from build123d import *

# Parameters (mm, degrees)
SKETCH1_W           = 25.25
SKETCH1_H           = 16
BOSS_EXTRUDE1_DEPTH = 1.7
BOSS_EXTRUDE3_DEPTH = 12.625
CUT_EXTRUDE7_DEPTH  = 9.75
CUT_EXTRUDE8_REACH  = 21.549


with BuildPart() as part:
    # Sketch1 → Boss-Extrude1 (new body)
    with BuildSketch(Plane(origin=(0, 0, 0), x_dir=(1, 0, 0), z_dir=(0, 1, 0))):
        Rectangle(SKETCH1_W, SKETCH1_H)
    extrude(amount=BOSS_EXTRUDE1_DEPTH)

    # Sketch5 → Boss-Extrude3 (add, symmetric)
    with BuildSketch(Plane(origin=(0, 0, 0), x_dir=(0, 0, -1), z_dir=(1, 0, 0))):
        Polygon((-8, 1.7), (8, 1.7), (8, 12.6), (5, 12.6), (-8, 5), align=None)
    extrude(amount=BOSS_EXTRUDE3_DEPTH, both=True)

    # Sketch5<2> → Cut-Extrude7 (cut, symmetric)
    with BuildSketch(Plane(origin=(0, 0, 0), x_dir=(0, 0, -1), z_dir=(1, 0, 0))):
        Polygon((-8, 1.7), (8, 1.7), (8, 12.6), (5, 12.6), (-8, 5), align=None)
    extrude(amount=CUT_EXTRUDE7_DEPTH, both=True, mode=Mode.SUBTRACT)

    # Sketch6 → Cut-Extrude8 (cut, up to next)
    with BuildSketch(Plane(origin=(0, 0, 0), x_dir=(1, 0, 0), z_dir=(0, 1, 0)), mode=Mode.PRIVATE) as cut_extrude8_sk1:
        with BuildLine():
            Line((-5.125, -2.5), (-2.325, -2.5))
            ThreePointArc((-2.325, -2.5), (-0.825, -4), (-2.325, -5.5))
            Line((-2.325, -5.5), (-5.125, -5.5))
            ThreePointArc((-5.125, -5.5), (-6.625, -4), (-5.125, -2.5))
        make_face()
    cut_extrude8_tool1 = extrude(cut_extrude8_sk1.sketch, amount=CUT_EXTRUDE8_REACH, mode=Mode.PRIVATE) & part.part
    # Sketch6 → Cut-Extrude8 (cut, up to next)
    with BuildSketch(Plane(origin=(0, 0, 0), x_dir=(1, 0, 0), z_dir=(0, 1, 0)), mode=Mode.PRIVATE) as cut_extrude8_sk2:
        with BuildLine():
            Line((2.325, 0), (5.125, 0))
            ThreePointArc((5.125, 0), (6.625, 1.5), (5.125, 3))
            Line((5.125, 3), (2.325, 3))
            ThreePointArc((2.325, 3), (0.825, 1.5), (2.325, 0))
        make_face()
    cut_extrude8_tool2 = extrude(cut_extrude8_sk2.sketch, amount=CUT_EXTRUDE8_REACH, mode=Mode.PRIVATE) & part.part
    add(cut_extrude8_tool1.solids().sort_by_distance((-3.725, 0, 4))[0], mode=Mode.SUBTRACT)
    add(cut_extrude8_tool2.solids().sort_by_distance((3.725, 0, -1.5))[0], mode=Mode.SUBTRACT)


solid = part.part
Model file for the job. Use its own axes, mm. A direction names the side the tool comes from. Coordinates: 2 decimals unless noted, no trailing zeros. Loops run counter-clockwise (first coordinate to the right, second up) from the corner with the lowest first, then second, coordinate; pieces in that order, holes last. Notation, with made-up numbers: (-36, 31) -> (5, 31) arc R18 cw to (5, 44) -> close; hole circle Ø9 at (31.5, 13). An arc over 180 degrees is marked (long way). Use one line per item in the form item = value. Start each with the question number.
(1) Cut at D-D on x = 8.75. Give the cut face in (y, z).
(2) Flat gauge pins, fed straight in: pin 1 (4 mm diameter, centred on x = 9, y = 11, fed in from +Z); pin 2 (5 mm diameter, centred on x = 9.5, z = 3.5, fed in from +Y) (3 decimals); pin 3 (5.5 mm diameter, centred on y = 9, z = 1.5, fed in from -X) (3 decimals); pin 4 (3 mm diameter, centred on x = -1, y = 3.5, fed in from +Z). Where does each tip first touch, or does it go through?
(3) Cut at B-B on z = 4. Give the cut face in (x, y) (3 decimals).
(4) Probe probe 1 along X at (y, z) = (3, -1.75) (3 decimals); probe 2 along Y at (x, z) = (-2.25, 1); probe 3 along Z at (x, y) = (-2, 1.25). List the from-to ranges inside material, lowest first. Write a range as from..to.
(5) Tool access for faces 1 (the cylindrical face through (0.825, 0.838, -1.533)), 2 (the flat face through (11.208, 8.853, 1.409)), 3 (the flat face through (9.75, 6, -2)): list every direction of +Z, -Z, +X, -X, +Y, -Y with a clear straight run to the whole face (end or side of a thin tool).
(6) Cut at A-A on x = 3.5. Give the cut face in (y, z), and give its area (3 significant figures).
(7) Pull direction X, two halves, no side cores. Call faces 4 (the flat face through (11, 12.6, -7)), 5 (the flat face through (-12.625, 5, -2)), 6 (the flat face through (-9.75, 6, -2)): pulls with the +X half, pulls with the -X half, needs draft (parallel to the pull), parting line crosses it, or undercut.
(8) Cut at C-C on z = -4.25. Give the cut face in (x, y) (3 decimals), and give its area (3 significant figures).
Values:
q1.outline = (0, -8) -> (1.7, -8) -> (1.7, 8) -> (0, 8) -> close
q2.pin_1 = 0.91
q2.pin_2 = 9.085
q2.pin_3 = -12.625
q2.pin_4 = through
q3.outline = (-12.625, 0) -> (-6.625, 0) -> (-6.625, 1.7) -> (-9.75, 1.7) -> (-9.75, 7.338) -> (-12.625, 7.338) -> close; (-0.825, 0) -> (12.625, 0) -> (12.625, 7.338) -> (9.75, 7.338) -> (9.75, 1.7) -> (-0.825, 1.7) -> close
q4.probe_1 = -12.625..-9.75, 9.75..12.625
q4.probe_2 = 0..1.7
q4.probe_3 = -8..2.54, 5.46..8
q5.face_1 = +Y, -Y
q5.face_2 = +Z, +X, -X, +Y
q5.face_3 = +Z, -Z, +Y
q6.outline = (0, -8) -> (1.7, -8) -> (1.7, -3) -> (0, -3) -> close; (0, 0) -> (1.7, 0) -> (1.7, 8) -> (0, 8) -> close
q6.area = 22.1 mm2
q7.face_4 = needs draft
q7.face_5 = pulls with the -X half
q7.face_6 = undercut
q8.outline = (-12.625, 0) -> (12.625, 0) -> (12.625, 12.162) -> (9.75, 12.162) -> (9.75, 1.7) -> (-9.75, 1.7) -> (-9.75, 12.162) -> (-12.625, 12.162) -> close
q8.area = 103 mm2
